Could you check a few things on this model? Use its own coordinates, in mm. A direction names the side the tool comes from. Round coordinates to 2 decimals unless told otherwise and drop trailing zeros. Write each loop counter-clockwise with the first axis right and the second up, starting at its lowest first coordinate (ties: lowest second). Pieces come first, ordered by that corner, then holes. Notation, with made-up numbers: (16.25, -8) - (51.25, -8) arc R13 ccw to (51.25, 3) - close; hole circle Ø5 at (-38.75, 85.25). An arc over 180 degrees is marked (long way). Put each result on its own line as item: value.
from build123d import *

# Parameters (mm, degrees)
SKETCH_1_W          = 10
SKETCH_1_H          = 10
SKETCH_1_W_2        = 8
SKETCH_1_H_2        = 8
EXTRUDE_1_DEPTH     = 340
SKETCH_2_R          = 1.5
CUT_EXTRUDE_1_DEPTH = 30
SKETCH_3_R          = 1.5
CUT_EXTRUDE_2_DEPTH = 10


with BuildPart() as part:
    # 草图1 → 凸台-拉伸1 (new body)
    with BuildSketch(Plane(origin=(0, 0, 0), x_dir=(1, 0, 0), z_dir=(0, 1, 0))):
        Rectangle(SKETCH_1_W, SKETCH_1_H)
        Rectangle(SKETCH_1_W_2, SKETCH_1_H_2, mode=Mode.SUBTRACT)
    extrude(amount=EXTRUDE_1_DEPTH)

    # 草图2 → 切除-拉伸1 (cut)
    with BuildSketch(Plane.ZY.offset(5)):
        with Locations((0, 5)):
            Circle(SKETCH_2_R)
        with Locations((0, 15)):
            Circle(SKETCH_2_R)
        with Locations((0, 225)):
            Circle(SKETCH_2_R)
        with Locations((0, 235)):
            Circle(SKETCH_2_R)
        with Locations((0, 245)):
            Circle(SKETCH_2_R)
        with Locations((0, 255)):
            Circle(SKETCH_2_R)
        with Locations((0, 265)):
            Circle(SKETCH_2_R)
    extrude(amount=-CUT_EXTRUDE_1_DEPTH, mode=Mode.SUBTRACT)

    # 草图3 → 切除-拉伸2 (cut)
    with BuildSketch(Plane(origin=(0, 0, -5), x_dir=(-1, 0, 0), z_dir=(0, 0, -1))):
        with Locations((0, 280)):
            Circle(SKETCH_3_R)
        with Locations((0, 330)):
            Circle(SKETCH_3_R)
    extrude(amount=-CUT_EXTRUDE_2_DEPTH, mode=Mode.SUBTRACT)


solid = part.part
(1) Please list where these lines run through material, in increasing order: probe 1 along Y at (x, z) = (0, 4.45); probe 2 along Z at (x, y) = (-2.25, 77); probe 3 along Z at (x, y) = (4.7, 225). Write a range as from..to.
Values found:
probe 1: y = 0..278.5, 281.5..328.5, 331.5..340
probe 2: z = -5..-4, 4..5
probe 3: z = -5..-1.5, 1.5..5
(2) For faces 1 (the face through (-4.5, 340, -0.1)), 2 (the face through (0, 168, -4)), which set-ups out of +Z, -Z, +X, -X, +Y, -Y let a thin tool reach every point of the face, with its end or its side?
Values found:
face 1: +Z, -Z, +X, -X, +Y
face 2: +Y, -Y
(3) Imagine slicing it at B-B, the plane y = 76.5. List the corners of the cut face in (x, z) for me.
Values found:
outline: (-5, -5) - (5, -5) - (5, 5) - (-5, 5) - close; hole (-4, -4) - (4, -4) - (4, 4) - (-4, 4) - close
(4) I'm going to push a flat-ended pin straight in: pin 1 (2.5 mm diameter, centred on y = 5, z = 0, fed in from +X). Where does the tip first touch, or does it pass through?
Values found:
pin 1: passes through
(5) If we mould it in two halves opening along X, with no side actions, what happens to faces 3 (the face through (-4, 168, 0)), 4 (the face through (-4.5, 0, -0.1)), 5 (the face through (5, 168, 0)), 6 (the face through (-5, 168, 0))? For each: pulls with the +X half, pulls with the -X half, needs draft (parallel to the pull), parting line crosses it, or undercut.
Values found:
face 3: undercut
face 4: needs draft
face 5: pulls with the +X half
face 6: pulls with the -X half
(6) Imagine slicing it at C-C, the plane z = 0. Give the number of separate pieces and of enclosed holes in the cut face, then the cut area to 3 significant figures.
Values found:
separate pieces: 16
enclosed holes: 0
area: 638 mm^2
(7) Imagine slicing it at A-A, the plane x = 0. List the corners of the cut face in (y, z) for me.
Values found:
outline: (0, -5) - (278.5, -5) - (278.5, -4) - (0, -4) - close; (0, 4) - (278.5, 4) - (278.5, 5) - (0, 5) - close; (281.5, -5) - (328.5, -5) - (328.5, -4) - (281.5, -4) - close; (281.5, 4) - (328.5, 4) - (328.5, 5) - (281.5, 5) - close; (331.5, -5) - (340, -5) - (340, -4) - (331.5, -4) - close; (331.5, 4) - (340, 4) - (340, 5) - (331.5, 5) - close
